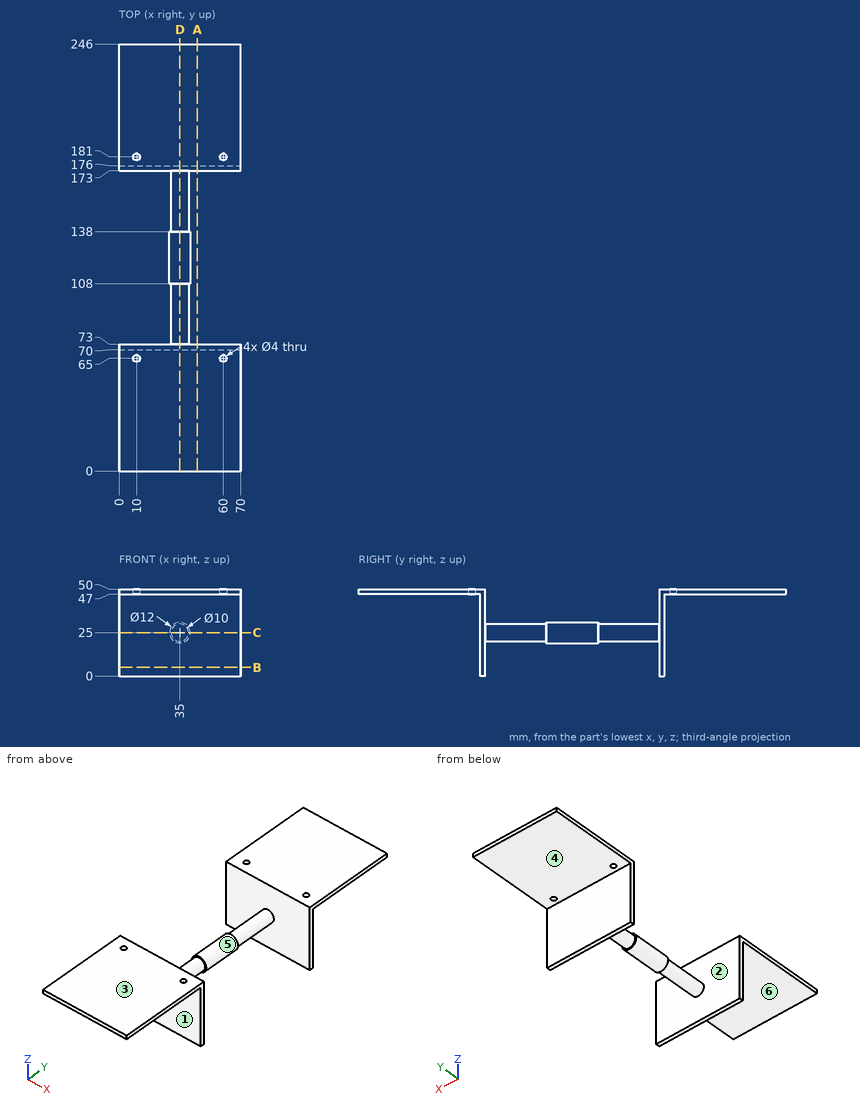
Source: three-view drawing plus pictorial views. Frame: mm from the lowest corner of the part. A direction names the side the tool comes from. Coordinates: 2 decimals unless noted, no trailing zeros. Write each loop counter-clockwise with the first axis right and the second up, starting at its lowest first coordinate (ties: lowest second). Pieces come first, ordered by that corner, then holes. Notation, with made-up numbers: (53.25, -35) -> (94.25, -35) arc R20 cw to (94.25, -1) -> close; hole circle Ø7 at (6.5, 83.25). An arc over 180 degrees is marked (long way). Write each question's results on one line, items separated by ' | '.
Item 1: Section query A-A on x = 45. Return loops of the section in (y, z), plus the area to 3 significant figures.
Conclusion:
outline: (0, 47) -> (70, 47) -> (70, 0) -> (73, 0) -> (73, 50) -> (0, 50) -> close; (173, 0) -> (176, 0) -> (176, 47) -> (246, 47) -> (246, 50) -> (173, 50) -> close | area: 720 mm^2
Item 2: Set-up query: the marked faces 4, 5 and 6. Return all of +Z, -Z, +X, -X, +Y, -Y with unobstructed straight access to the full face (end or side cutting, diameter ignored); none if empty.
Conclusion:
face 4: -Z, +X, -X, +Y | face 5: none | face 6: -Z, +X, -X, -Y
Item 3: Section query D-D on x = 35. Return loops of the section in (y, z).
Conclusion:
outline: (0, 47) -> (70, 47) -> (70, 0) -> (73, 0) -> (73, 20) -> (108, 20) -> (108, 19) -> (138, 19) -> (138, 20) -> (173, 20) -> (173, 0) -> (176, 0) -> (176, 47) -> (246, 47) -> (246, 50) -> (173, 50) -> (173, 30) -> (138, 30) -> (138, 31) -> (108, 31) -> (108, 30) -> (73, 30) -> (73, 50) -> (0, 50) -> close
Item 4: Pin query (flat end, axial travel): pin 1 Ø6 at (x, z) = (41.5, 43.5) entering from -Y; pin 2 Ø2 at (x, z) = (19, 32) entering from +Y; pin 3 Ø3 at (x, y) = (10, 181) entering from +Z; pin 4 Ø8 at (x, y) = (31, 194.5) entering from -Z. Return the tip coordinate at first contact, or that it passes through.
Conclusion:
pin 1: stops at y = 70 | pin 2: stops at y = 176 | pin 3: passes through | pin 4: stops at z = 47
Item 5: Section query B-B on z = 5. Return loops of the section in (x, y), plus the area to 3 significant figures.
Conclusion:
outline: (0, 70) -> (70, 70) -> (70, 73) -> (0, 73) -> close; (0, 173) -> (70, 173) -> (70, 176) -> (0, 176) -> close | area: 420 mm^2
Item 6: Section query C-C on z = 25. Return loops of the section in (x, y).
Conclusion:
outline: (0, 70) -> (70, 70) -> (70, 73) -> (40, 73) -> (40, 108) -> (41, 108) -> (41, 138) -> (40, 138) -> (40, 173) -> (70, 173) -> (70, 176) -> (0, 176) -> (0, 173) -> (30, 173) -> (30, 138) -> (29, 138) -> (29, 108) -> (30, 108) -> (30, 73) -> (0, 73) -> close
Item 7: Mould query, pull axis Y, two halves, no side actions, for the marked faces 1, 2 and 3. Classes: +Y half, -Y half, draft (parallel to the pull), parting line (faces both ways), or undercut.
Conclusion:
face 1: -Y half | face 2: undercut | face 3: draft
Item 8: Material intervals for probe 1 along X at (y, z) = (181, 48.4); probe 2 along Y at (x, z) = (10, 49.25); probe 3 along Y at (x, z) = (14, 41), sorted ascending.
Conclusion:
probe 1: x = 0 to 8, 12 to 58, 62 to 70 | probe 2: y = 0 to 63, 67 to 73, 173 to 179, 183 to 246 | probe 3: y = 70 to 73, 173 to 176
